Autodesk Inventor part; units mm, degrees
ref_plane "YZ Plane" through (0, 0, 0) normal (1, 0, 0) x (0, 1, 0)
ref_plane "XZ Plane" through (0, 0, 0) normal (0, 1, 0) x (-1, 0, 0)
ref_plane "XY Plane" through (0, 0, 0) normal (0, 0, 1) x (1, 0, 0)
sketch "Sketch1" plane through (0, 0, 0) normal (0, 0, 1) x (1, 0, 0)
  line L0 (0, 0) -> (25, 0)
  line L1 (25, 0) -> (25, 10)
  line L2 (25, 10) -> (0, 10)
  line L3 (0, 10) -> (0, 0)
  dimension "d0" = 25
  dimension "d1" = 10
extrude "Extrusion1" add sketch "Sketch1" along normal blind 2
fillet "Fillet1" radius 5 4 edges at (25, 10, 1) (25, 0, 1) (0, 0, 1) (0, 10, 1)
sketch "Sketch2" plane through (0, 0, 2) normal (0, 0, 1) x (1, 0, 0)
  arc A0 (5, 10) -> (5, 0) centre (5, 5) ccw
  arc A1 (20, 0) -> (20, 10) centre (20, 5) ccw
  line L0 (5, 5) -> (4, 5)
  line L1 (4, 5) -> (21, 5)
  circle A2 centre (4, 5) radius 1.5
  circle A3 centre (21, 5) radius 1.5
  point P0 (0, 0)
  dimension "d9" = 1
  dimension "d10" = 17
  dimension "d11" = 3
  dimension "d12" = 3
extrude "Extrusion3" cut sketch "Sketch2" against normal blind 10
properties part number "Middle support"
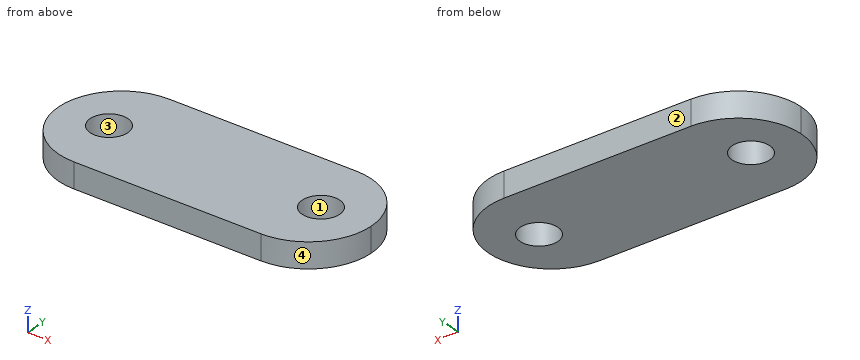
CAD build for the part. Positions are in the model's coordinates, mm. Face numbers are marked on the shaded views. Give positions to 0.01 mm unless a question says otherwise; leave off trailing zeros. Loops run counter-clockwise (first coordinate to the right, second up) from the corner with the lowest first, then second, coordinate; pieces in that order, holes last. Notation, with made-up numbers: (28.25, 56.5) -> (59.25, 56.5) arc R29 ccw to (59.25, 80.5) -> close; hole circle Ø1 at (6, -22.75). An arc over 180 degrees is marked (long way). Use a Markdown table: item, result.
1. Flat gauge pin, fed straight in: pin 1 (1 mm diameter, centred on y = 6.5, z = 1, fed in from +X). Where does the tip first touch, or does it go through?
Check result:
| item | result |
|---|---|
| pin 1 | stops at x = 24.9 |
2. Slice it at B-B (z = 1.35). Give the number of separate pieces and of enclosed holes in the cut face, plus the area to 3 significant figures.
Check result:
| item | result |
|---|---|
| separate pieces | 1 |
| enclosed holes | 2 |
| area | 214 mm^2 |
3. Wall check: L1, parallel to X at y = 5.5, z = 1.1; L2, parallel to X at y = 4.25, z = 1.7; L3, parallel to Y at x = 21.75, z = 1.2. Give the ranges that are in metal, low to high. Write a range as [from, to].
Check result:
| item | result |
|---|---|
| L1 | x = [0.03, 2.59], [5.41, 19.59], [22.41, 24.97] |
| L2 | x = [0.06, 2.7], [5.3, 19.7], [22.3, 24.94] |
| L3 | y = [0.32, 3.7], [6.3, 9.68] |
4. Mould opens along X. For the marked faces 1, 2, 3 and 4 say: pulls with the +X half, pulls with the -X half, needs draft (parallel to the pull), parting line crosses it, or undercut.
Check result:
| item | result |
|---|---|
| face 1 | undercut |
| face 2 | needs draft |
| face 3 | undercut |
| face 4 | pulls with the +X half |
5. Slice it at C-C (x = 21). List the corners of the cut face in (y, z), plus the area to 3 significant figures.
Check result:
| item | result |
|---|---|
| outline | (0.1, 0) -> (3.5, 0) -> (3.5, 2) -> (0.1, 2) -> close; (6.5, 0) -> (9.9, 0) -> (9.9, 2) -> (6.5, 2) -> close |
| area | 13.6 mm^2 |
6. Slice it at A-A (y = 3.75). List the corners of the cut face in (x, z).
Check result:
| item | result |
|---|---|
| outline | (0.16, 0) -> (3.17, 0) -> (3.17, 2) -> (0.16, 2) -> close; (4.83, 0) -> (20.17, 0) -> (20.17, 2) -> (4.83, 2) -> close; (21.83, 0) -> (24.84, 0) -> (24.84, 2) -> (21.83, 2) -> close |
